Part model, mm, in its own coordinate system. Face numbers are marked on the shaded views. A direction names the side the tool comes from. Round coordinates to 2 decimals unless told otherwise and drop trailing zeros. Loops run counter-clockwise (first coordinate to the right, second up) from the corner with the lowest first, then second, coordinate; pieces in that order, holes last. Notation, with made-up numbers: (9, 66) -> (56, 66) arc R26 cw to (56, 94) -> close; hole circle Ø2 at (-35, -25). An arc over 180 degrees is marked (long way). Use a Markdown table: item, result. Add a question column.
Item 1: Flat gauge pin, fed straight in: pin 1 (9 mm diameter, centred on x = -16, y = 1.5, fed in from +Z). Where does the tip first touch, or does it go through?
Item 2: Probe line 1 (Z direction, x = 17, y = 2); line 2 (Y direction, x = 20, z = 22.75); line 3 (Y direction, x = 29.5, z = 16.5). List the from-to ranges inside material, lowest first. Write a range as [from, to].
Item 3: Which spindle directions (+Z, -Z, +X, -X, +Y, -Y) get a long thin tool onto all of the face, cutting with end or side? Do the marked faces 1 and 2. Say none if no direction does.
Item 4: Cut at A-A, the plane z = 20. List the corners of the cut face in (x, y).
Item 5: Two-plate mould, pull along Y, no slides. Class the marked faces 3, 4 and 5: pulls with the +Y half, pulls with the -Y half, needs draft (parallel to the pull), parting line crosses it, or undercut.
Item 6: Cut at B-B, the plane x = -18. List the corners of the cut face in (y, z).
Item 7: Cut at C-C, the plane y = 2. List the corners of the cut face in (x, z).
Item 8: Cut at D-D, the plane y = 13.5. List the corners of the cut face in (x, z).
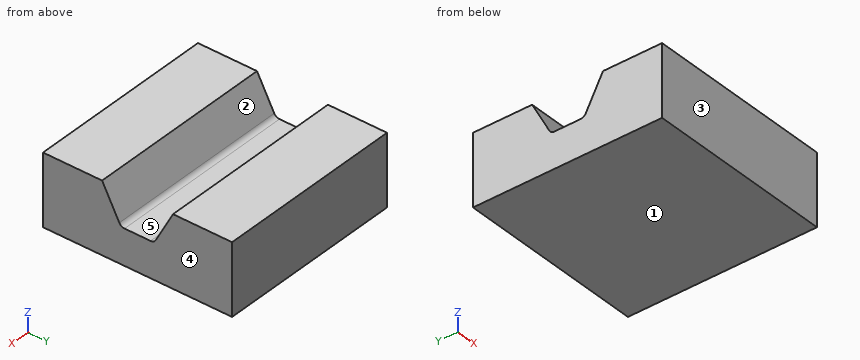
```python
from build123d import *

# Parameters (mm, degrees)
CROQUIS1_W              = 80
CROQUIS1_H              = 80
SALIENTE_EXTRUIR1_DEPTH = 30
CORTAR_EXTRUIR1_DEPTH   = 95.339811321


with BuildPart() as part:
    # Croquis1 → Saliente-Extruir1 (new body)
    with BuildSketch(Plane.XY):
        Rectangle(CROQUIS1_W, CROQUIS1_H)
    extrude(amount=SALIENTE_EXTRUIR1_DEPTH)

    # Croquis2 → Cortar-Extruir1 (cut, through all)
    with BuildSketch(Plane(origin=(40, 0, 0), x_dir=(0, 0, -1), z_dir=(1, 0, 0))):
        with BuildLine():
            Line((-30, 15), (-16.323529412, 7.705882353))
            ThreePointArc((-16.323529412, 7.705882353), (-15.356267686, 6.786239389), (-15, 5.5))
            Line((-15, 5.5), (-15, -5.5))
            ThreePointArc((-15, -5.5), (-15.356267686, -6.786239389), (-16.323529412, -7.705882353))
            Line((-16.323529412, -7.705882353), (-30, -15))
            Line((-30, -15), (-30, 15))
        make_face()
    extrude(amount=-CORTAR_EXTRUIR1_DEPTH, mode=Mode.SUBTRACT)


solid = part.part
```
A:
| question | item | result |
|---|---|---|
| 1 | pin 1 | stops at z = 15.05 |
| 2 | line 1 | z = [0, 15] |
| 2 | line 2 | y = [-40, -11.13], [11.13, 40] |
| 2 | line 3 | y = [-40, -7.8], [7.8, 40] |
| 3 | face 1 | -Z, +X, -X, +Y, -Y |
| 3 | face 2 | +Z, +X, -X |
| 4 | outline | (-40, -40) -> (40, -40) -> (40, -9.67) -> (-40, -9.67) -> close; (-40, 9.67) -> (40, 9.67) -> (40, 40) -> (-40, 40) -> close |
| 5 | face 3 | pulls with the -Y half |
| 5 | face 4 | needs draft |
| 5 | face 5 | undercut |
| 6 | outline | (-40, 0) -> (40, 0) -> (40, 30) -> (15, 30) -> (7.71, 16.32) arc R2.5 cw to (5.5, 15) -> (-5.5, 15) arc R2.5 cw to (-7.71, 16.32) -> (-15, 30) -> (-40, 30) -> close |
| 7 | outline | (-40, 0) -> (40, 0) -> (40, 15) -> (-40, 15) -> close |
| 8 | outline | (-40, 0) -> (40, 0) -> (40, 27.19) -> (-40, 27.19) -> close |
